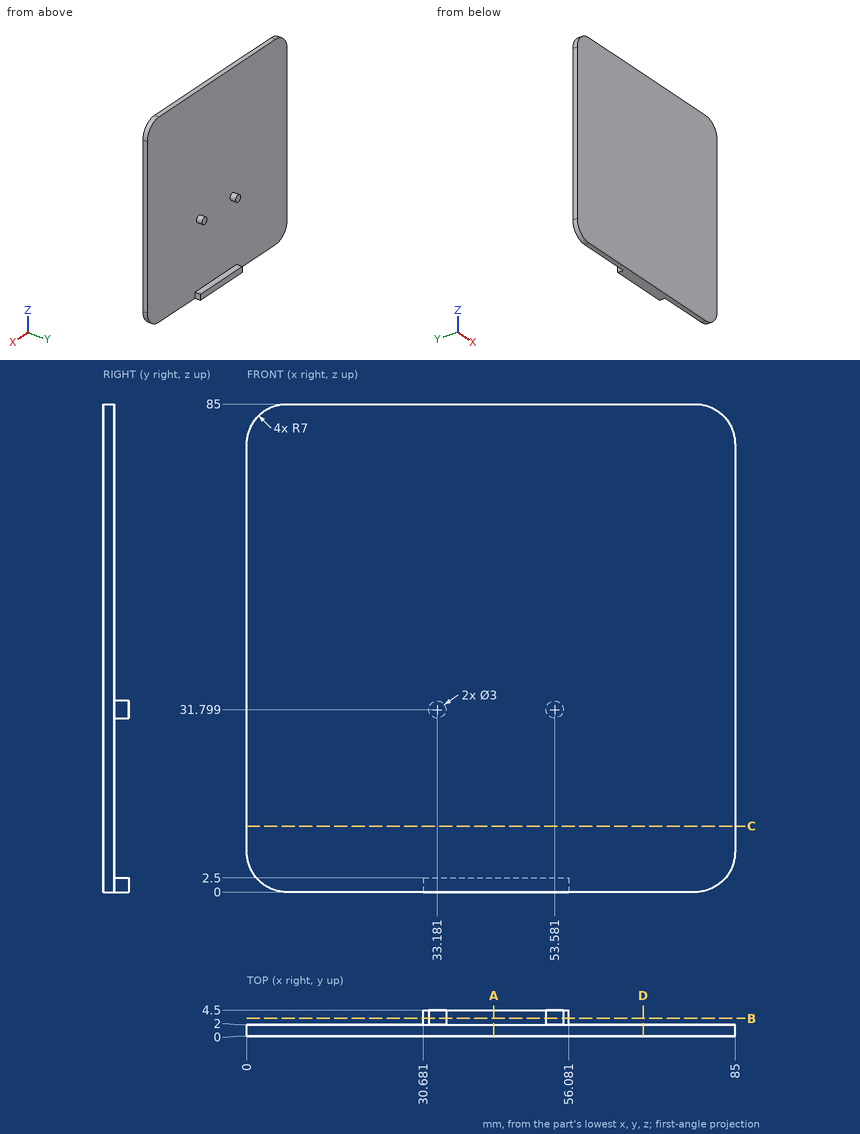
Design review of the part shown in the three views and the two pictorial views. Dimensions are in mm from the part's minimum x, y and z. Give positions to 0.01 mm unless a question says otherwise; leave off trailing zeros. Write each loop counter-clockwise with the first axis right and the second up, starting at its lowest first coordinate (ties: lowest second). Pieces come first, ordered by that corner, then holes.
Item 1: Take a section at D-D (x = 69). Give the boundary of the cut face in (y, z).
Item 2: Wall thickness on probe 1 along Y at (x, z) = (75, 52.5); probe 2 along Z at (x, y) = (38, 3.25); probe 3 along Z at (x, y) = (34, 3.1) (1 decimal): over which ranges is each line inside the solid? List them lowest first.
Item 3: Take a section at A-A (x = 43). Give the boundary of the cut face in (y, z).
Item 4: Take a section at C-C (z = 11.5). Give the boundary of the cut face in (x, y).
Item 5: Take a section at B-B (y = 3.05). Give the boundary of the cut face in (x, z).
Item 6: Insertion check: P1, Ø12, axis at x = 32.5, z = 52.5, coming from the +Y side. The pin has a flat end and moves straight along its axis. Give the tip position at first contact, or say it passes through.
Established:
1. outline: (0, 0) - (2, 0) - (2, 85) - (0, 85) - close
2. probe 1: y = 0 to 2
2. probe 2: z = 0 to 2.5
2. probe 3: z = 0 to 2.5, 30.5 to 33.1
3. outline: (0, 0) - (4.5, 0) - (4.5, 2.5) - (2, 2.5) - (2, 85) - (0, 85) - close
4. outline: (0, 0) - (85, 0) - (85, 2) - (0, 2) - close
5. outline: (30.68, 0) - (56.08, 0) - (56.08, 2.5) - (30.68, 2.5) - close; circle Ø3 at (33.18, 31.8); circle Ø3 at (53.58, 31.8)
6. P1: stops at y = 2
